from build123d import *

# Parameters (mm, degrees)
BOSS_EXTRUDE1_DEPTH = 609.6
LPATTERN1_COUNT     = 12
LPATTERN1_PITCH     = 101.6


with BuildPart() as part:
    # Sketch1 → Boss-Extrude1 (new, symmetric)
    with BuildSketch(Plane.XY):
        Polygon((-4.7625, 0), (-9.525, 0), (-9.525, -9.525), (9.525, -9.525), (9.525, 0), (4.7625, 0), (4.7625, -2.38125), (7.14375, -2.38125), (7.14375, -4.7625), (5.55625, -4.7625), (5.55625, -7.14375), (-5.55625, -7.14375), (-5.55625, -4.7625), (-7.14375, -4.7625), (-7.14375, -2.38125), (-4.7625, -2.38125), align=None)
    extrude(amount=BOSS_EXTRUDE1_DEPTH, both=True)

    # Sketch7 → CSK for #6 Flat Head Machine Screw2 (revolve, cut)
    with BuildSketch(Plane(origin=(0, -7.14375, -558.8), x_dir=(0, 0, 1), z_dir=(1, 0, 0))):
        Polygon((0, 0), (0, 2.38125), (1.89865, 2.38125), (1.89865, 1.891953401), (3.5433, 0), align=None)
    csk_for_6_flat_head_machine_screw2 = revolve(axis=Axis((0, -0.79375, -558.8), (0, -1, 0)), mode=Mode.SUBTRACT)

    # LPattern1: CSK for #6 Flat Head Machine Screw2 ×12
    with Locations(*[(0, 0, i * LPATTERN1_PITCH) for i in range(1, LPATTERN1_COUNT)]):
        add(csk_for_6_flat_head_machine_screw2, mode=Mode.SUBTRACT)


solid = part.part
Design review of the part built by this model. Coordinates are the model's own, in mm. Coordinates: 2 decimals unless noted, no trailing zeros. Write each loop counter-clockwise with the first axis right and the second up, starting at its lowest first coordinate (ties: lowest second). Pieces come first, ordered by that corner, then holes. Notation, with made-up numbers: (4, 45.25) - (16, 45.25) arc R24 ccw to (16, 72.25) - close; hole circle Ø7 at (-18.75, 66.25). An arc over 180 degrees is marked (long way). One line per item, written item: value.
1) Add section A-A (z = 207). State the section outline as (x, y) points (1 decimal), plus the area to 3 significant figures.
Answer sheet:
outline: (-9.5, -9.5) - (9.5, -9.5) - (9.5, 0) - (4.8, 0) - (4.8, -2.4) - (7.1, -2.4) - (7.1, -4.8) - (5.6, -4.8) - (5.6, -7.1) - (-5.6, -7.1) - (-5.6, -4.8) - (-7.1, -4.8) - (-7.1, -2.4) - (-4.8, -2.4) - (-4.8, 0) - (-9.5, 0) - close
area: 98.3 mm2
2) Insertion check: pin 1 (3.5 mm diameter, centred on x = 0, z = -355.6, fed in from -Y); pin 2 (1.5 mm diameter, centred on x = -3.5, z = -138.5, fed in from +Y); pin 3 (4.5 mm diameter, centred on x = 0, z = 152.4, fed in from +Y). Each pin has a flat end and moves straight along its axis. Give the tip position at first contact, or say it passes through.
Answer sheet:
pin 1: passes through
pin 2: stops at y = -7.14
pin 3: stops at y = -8.63
3) To check wall thickness, follow probe 1 along X at (y, z) = (-6.5, 159.5) (3 decimals); probe 2 along Y at (x, z) = (-5.5, -44) (3 decimals); probe 3 along X at (y, z) = (-4, -119) (3 decimals). State the ranges of each line that lie inside material, in increasing order.
Answer sheet:
probe 1: x = -9.525 to -5.556, 5.556 to 9.525
probe 2: y = -9.525 to -7.144, -2.381 to 0
probe 3: x = -9.525 to -7.144, 7.144 to 9.525
